Read the model definition and answer for the solid it produces. Units are mm, in the model's axes. Face numbers are marked on the shaded views. A direction names the side the tool comes from. Coordinates: 2 decimals unless noted, no trailing zeros. Write each loop counter-clockwise with the first axis right and the second up, starting at its lowest first coordinate (ties: lowest second). Pieces come first, ordered by that corner, then holes.
(1) Which of the six approach directions +Z, -Z, +X, -X, +Y, -Y give full straight-line access (tool end or side, diameter ignored) to the marked faces 1 and 2?
(2) Section D-D on z = -5.75 is taken. Write down the section's boundary in (x, y), then the cut area to 3 significant figures.
(3) Find the intervals of material crossed by probe 1 along Z at (x, y) = (0.25, 45); probe 2 along X at (y, z) = (67.5, 0); probe 3 along Y at (x, z) = (-1.5, -6.5), in increasing order.
(4) Section B-B on z = 0 is taken. Write down the section's boundary in (x, y), then the cut area to 3 significant figures.
(5) Section C-C on y = 56 is taken. Write down the section's boundary in (x, z).
(6) Section A-A on x = 0 is taken. Write down the section's boundary in (y, z), then the cut area to 3 significant figures.
(7) Given pin 1 (1.2 mm diameter, centred on x = -1, y = 156.5, fed in from +Z); pin 2 (1.5 mm diameter, centred on x = -0.5, z = 0, fed in from +Y); pin 3 (4 mm diameter, centred on x = -3, y = 74.5, fed in from -Z); pin 4 (5 mm diameter, centred on y = 122.5, z = -4, fed in from +X), each flat-ended and moving along its own axis, determine where each tip first touches the part or whether it passes through.
from build123d import *

# Parameters (mm, degrees)
SKETCH1_R           = 4.25
BOSS_EXTRUDE1_DEPTH = 7.9
SKETCH2_R           = 7.5
BOSS_EXTRUDE2_DEPTH = 150
SKETCH3_R           = 2.25
CUT_EXTRUDE1_DEPTH  = 159.255837175
SKETCH4_W           = 15
SKETCH4_H           = 5
CUT_EXTRUDE2_DEPTH  = 2.5


with BuildPart() as part:
    # Sketch1 → Boss-Extrude1 (new body)
    with BuildSketch(Plane(origin=(0, 0, 0), x_dir=(1, 0, 0), z_dir=(0, 1, 0))):
        with Locations(Location((0, 0, 0), (0, 0, 270))):
            Circle(SKETCH1_R)
    extrude(amount=BOSS_EXTRUDE1_DEPTH)

    # Sketch2 → Boss-Extrude2 (add)
    with BuildSketch(Plane(origin=(0, 7.9, 0), x_dir=(1, 0, 0), z_dir=(0, 1, 0))):
        with Locations(Location((0, 0, 0), (0, 0, 270))):
            Circle(SKETCH2_R)
    extrude(amount=BOSS_EXTRUDE2_DEPTH)

    # Sketch3 → Cut-Extrude1 (cut, through all)
    with BuildSketch(Plane(origin=(0, 157.9, 0), x_dir=(1, 0, 0), z_dir=(0, 1, 0))):
        with Locations(Location((0, 0, 0), (0, 0, 270))):
            Circle(SKETCH3_R)
    extrude(amount=-CUT_EXTRUDE1_DEPTH, mode=Mode.SUBTRACT)

    # Sketch4 → Cut-Extrude2 (cut)
    with BuildSketch(Plane(origin=(0, 157.9, 0), x_dir=(1, 0, 0), z_dir=(0, 1, 0))):
        Rectangle(SKETCH4_W, SKETCH4_H)
    extrude(amount=-CUT_EXTRUDE2_DEPTH, mode=Mode.SUBTRACT)


solid = part.part
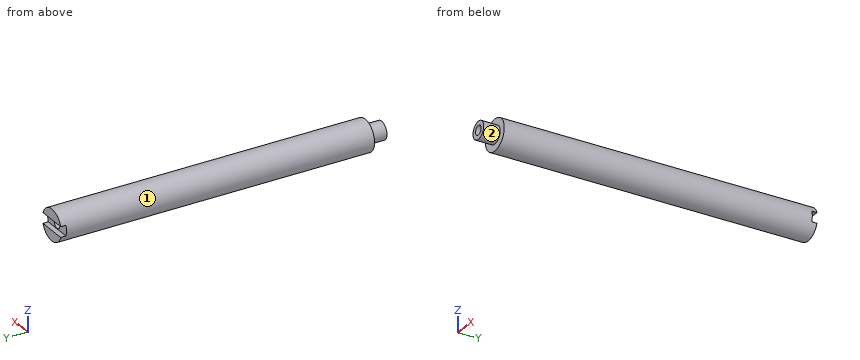
Response:
1. face 1: +Y, -Y
1. face 2: -Y
2. outline: (-4.82, 7.9) - (4.82, 7.9) - (4.82, 157.9) - (-4.82, 157.9) - close
2. area: 1,440 mm2
3. probe 1: z = -7.5 to -2.24, 2.24 to 7.5
3. probe 2: x = -7.5 to -2.25, 2.25 to 7.5
3. probe 3: y = 7.9 to 157.9
4. outline: (-7.5, 7.9) - (-4.25, 7.9) - (-4.25, 0) - (-2.25, 0) - (-2.25, 155.4) - (-7.5, 155.4) - close; (2.25, 0) - (4.25, 0) - (4.25, 7.9) - (7.5, 7.9) - (7.5, 155.4) - (2.25, 155.4) - close
4. area: 1,580 mm2
5. outline: circle Ø15 at (0, 0); hole circle Ø4.5 at (0, 0)
6. outline: (0, -4.25) - (7.9, -4.25) - (7.9, -7.5) - (157.9, -7.5) - (157.9, -2.5) - (155.4, -2.5) - (155.4, -2.25) - (0, -2.25) - close; (0, 2.25) - (155.4, 2.25) - (155.4, 2.5) - (157.9, 2.5) - (157.9, 7.5) - (7.9, 7.5) - (7.9, 4.25) - (0, 4.25) - close
6. area: 1,610 mm2
7. pin 1: stops at z = 7.49
7. pin 2: passes through
7. pin 3: stops at z = -7.43
7. pin 4: stops at x = 7.35
